Work out the finished part from the listing and answer in its coordinate system (mm). A direction names the side the tool comes from. Give positions to 0.01 mm unless a question says otherwise; leave off trailing zeros. Write each loop counter-clockwise with the first axis right and the second up, starting at its lowest first coordinate (ties: lowest second). Pieces come first, ordered by that corner, then holes. Notation, with made-up numbers: (4.5, 87.25) -> (35.5, 87.25) arc R6 ccw to (35.5, 95.25) -> close; hole circle Ø8 at (-24, 45). An arc over 180 degrees is marked (long way). Use a Markdown table: item, result. Add a question column.
Q1. For a pull along X with two mould halves and no side action, classify faces 1 (the face through (-9.715, 3.324, -9.699)), 2 (the face through (-6.1, 10, 2.1)), 3 (the face through (-9, 5, 0)), 4 (the face through (9, 5, 0)) as pulls with the +X half, pulls with the -X half, needs draft (parallel to the pull), parting line crosses it, or undercut.
Q2. Consider line 1 (X direction, y = 1.25, z = 0); line 2 (X direction, y = -6.55, z = 0); line 3 (Z direction, x = -4.25, y = 0). Determine where each line is inside the solid, lowest interval first.
Q3. For faces 5 (the face through (-9.5, 0, 0.1)), 6 (the face through (1.88, 4.08, 5.96)), 7 (the face through (9.5, 0, 0.1)), 8 (the face through (0.1, 0, 9.5)), determine the directions among +Z, -Z, +X, -X, +Y, -Y from which every point of the face is accessible in a straight line to the end or side of a thin tool.
Q4. Each of these flat-tipped pins is pushed along its axis until it touches: pin 1 Ø4 at (x, z) = (1, 1.5) entering from +Y; pin 2 Ø8 at (x, y) = (5, -6) entering from +Z. Where does it stop, or does it pass through?
Q5. Section B-B, the plane z = 0 is taken. Give the vertices of the cut face in (x, y).
Q6. Section D-D, the plane y = -1.25 is taken. State how many separate pieces and enclosed holes the cut face has, plus the area to 3 significant figures.
Q7. Section A-A, the plane y = 2.25 is taken. Give the vertices of the cut face in (x, z).
Q8. Section C-C, the plane x = 0 is taken. Give the vertices of the cut face in (y, z).
from build123d import *

# Parameters (mm, degrees)
IZIM1_W                     = 20
IZIM1_H                     = 20
Y_KSEKLIK_EKSTR_ZYON1_DEPTH = 10
BO_ALTMA1_T                 = -1
IZIM2_R                     = 7
Y_KSEKLIK_EKSTR_ZYON2_DEPTH = 17
IZIM3_R                     = 20
KES_EKSTR_ZYON2_DEPTH       = 1
IZIM4_R                     = 20
KES_EKSTR_ZYON3_DEPTH       = 1
IZIM5_R                     = 6.25
KES_EKSTR_ZYON4_DEPTH       = 12
IZIM6_R                     = 3.25
KES_EKSTR_ZYON5_DEPTH       = 10
IZIM7_R                     = 8
IZIM7_R_2                   = 5
KES_EKSTR_ZYON6_DEPTH       = 5
RADYUS2_R                   = 1


with BuildPart() as part:
    # Çizim1 → Yükseklik-Ekstrüzyon1 (new, symmetric)
    with BuildSketch(Plane.XY):
        Rectangle(IZIM1_W, IZIM1_H)
    extrude(amount=Y_KSEKLIK_EKSTR_ZYON1_DEPTH, both=True)

    # İç Boşaltma1
    bo_altma1_openings = [part.faces().sort_by_distance(p)[0] for p in [
        (0, -10, 0),
    ]]
    offset(amount=BO_ALTMA1_T, openings=bo_altma1_openings, kind=Kind.INTERSECTION)

    # Çizim2 → Yükseklik-Ekstrüzyon2 (add)
    with BuildSketch(Plane.XZ.offset(-9)):
        with Locations(Location((0, 0, 0), (0, 0, 270))):
            Circle(IZIM2_R)
    extrude(amount=Y_KSEKLIK_EKSTR_ZYON2_DEPTH)

    # Çizim3 → Kes-Ekstrüzyon2 (cut)
    with BuildSketch(Plane.ZY.offset(10)):
        with Locations((0, -20)):
            Circle(IZIM3_R)
    kes_ekstr_zyon2 = extrude(amount=-KES_EKSTR_ZYON2_DEPTH, mode=Mode.SUBTRACT)

    # Aynalama1: Kes-Ekstrüzyon2 across plane
    add(kes_ekstr_zyon2.mirror(Plane(origin=(0, 0, 0), x_dir=(0, 0, 1), z_dir=(1, 0, 0))), mode=Mode.SUBTRACT)

    # Çizim4 → Kes-Ekstrüzyon3 (cut)
    with BuildSketch(Plane.XY.offset(10)):
        with Locations((0, -20)):
            Circle(IZIM4_R)
    kes_ekstr_zyon3 = extrude(amount=-KES_EKSTR_ZYON3_DEPTH, mode=Mode.SUBTRACT)

    # Aynalama2: Kes-Ekstrüzyon3 across plane
    add(kes_ekstr_zyon3.mirror(Plane.XY), mode=Mode.SUBTRACT)

    # Çizim5 → Kes-Ekstrüzyon4 (cut)
    with BuildSketch(Plane(origin=(0, 10, 0), x_dir=(1, 0, 0), z_dir=(0, 1, 0))):
        with Locations(Location((0, 0, 0), (0, 0, 270))):
            Circle(IZIM5_R)
    extrude(amount=-KES_EKSTR_ZYON4_DEPTH, mode=Mode.SUBTRACT)

    # Çizim6 → Kes-Ekstrüzyon5 (cut)
    with BuildSketch(Plane(origin=(0, -2, 0), x_dir=(1, 0, 0), z_dir=(0, 1, 0))):
        with Locations(Location((0, 0, 0), (0, 0, 270))):
            Circle(IZIM6_R)
    extrude(amount=-KES_EKSTR_ZYON5_DEPTH, mode=Mode.SUBTRACT)

    # Çizim7 → Kes-Ekstrüzyon6 (cut)
    with BuildSketch(Plane.XZ.offset(8)):
        Circle(IZIM7_R)
        with Locations(Location((0, 0, 0), (0, 0, 270))):
            Circle(IZIM7_R_2, mode=Mode.SUBTRACT)
    extrude(amount=-KES_EKSTR_ZYON6_DEPTH, mode=Mode.SUBTRACT)

    # Radyus2
    radyus2_edges = [part.edges().sort_by_distance(p)[0] for p in [
        (-10, 3.660254038, 10),
        (10, 3.660254038, -10),
        (10, 3.660254038, 10),
        (-10, 3.660254038, -10),
        (0, 10, -10),
        (0, 10, 10),
        (-10, 10, 0),
        (10, 10, 0),
    ]]
    fillet(radyus2_edges, radius=RADYUS2_R)


solid = part.part
Result set:
| question | item | result |
|---|---|---|
| 1 | face 1 | pulls with the -X half |
| 1 | face 2 | needs draft |
| 1 | face 3 | undercut |
| 1 | face 4 | undercut |
| 2 | line 1 | x = -10 to -9, -7 to -6.25, 6.25 to 7, 9 to 10 |
| 2 | line 2 | x = -5 to -3.25, 3.25 to 5 |
| 2 | line 3 | z = -10 to -9, -5.56 to -4.58, 4.58 to 5.56, 9 to 10 |
| 3 | face 5 | -X, -Y |
| 3 | face 6 | +Y |
| 3 | face 7 | +X, -Y |
| 3 | face 8 | +Z, -Y |
| 4 | pin 1 | stops at y = -2 |
| 4 | pin 2 | stops at z = 6.59 |
| 5 | outline | (-10, 0) -> (-9, 0) -> (-9, 9) -> (-7, 9) -> (-7, -3) -> (-5, -3) -> (-5, -8) -> (-3.25, -8) -> (-3.25, -2) -> (-6.25, -2) -> (-6.25, 10) -> (-9, 10) arc R1 ccw to (-10, 9) -> close; (3.25, -8) -> (5, -8) -> (5, -3) -> (7, -3) -> (7, 9) -> (9, 9) -> (9, 0) -> (10, 0) -> (10, 9) arc R1 ccw to (9, 10) -> (6.25, 10) -> (6.25, -2) -> (3.25, -2) -> close |
| 6 | separate pieces | 5 |
| 6 | enclosed holes | 1 |
| 6 | area | 50.7 mm2 |
| 7 | outline | (-10, -9) arc R1 ccw to (-9, -10) -> (9, -10) arc R1 ccw to (10, -9) -> (10, 9) arc R1 ccw to (9, 10) -> (-9, 10) arc R1 ccw to (-10, 9) -> close; circle Ø14 at (0, 0); hole (-9, -9) -> (9, -9) -> (9, 9) -> (-9, 9) -> close; hole circle Ø12.5 at (0, 0) |
| 8 | outline | (-8, -5) -> (-3, -5) -> (-3, -7) -> (9, -7) -> (9, -9) -> (0, -9) -> (0, -10) -> (9, -10) arc R1 ccw to (10, -9) -> (10, -6.25) -> (-2, -6.25) -> (-2, -3.25) -> (-8, -3.25) -> close; (-8, 3.25) -> (-2, 3.25) -> (-2, 6.25) -> (10, 6.25) -> (10, 9) arc R1 ccw to (9, 10) -> (0, 10) -> (0, 9) -> (9, 9) -> (9, 7) -> (-3, 7) -> (-3, 5) -> (-8, 5) -> close |
